Solid Edge part; units mm, degrees
sketch "Sketch1" plane through (0, 0, 0) normal (0, 0, 1) x (1, 0, 0)
  line L0 (-3, -3) -> (3, -3)
  line L1 (3, -3) -> (3, 3)
  line L2 (3, 3) -> (-3, 3)
  line L3 (-3, 3) -> (-3, -3)
extrude "Protrusion1" add sketch "Sketch1" along normal blind 2.5
sketch "Sketch2" plane through (0, 0, 2.5) normal (0, 0, 1) x (1, 0, 0)
  circle A0 centre (0, 0) radius 1
extrude "ExtrudedCutout_2" cut sketch "Sketch2" against normal blind 1
properties material "ABS Plastic, high impact"
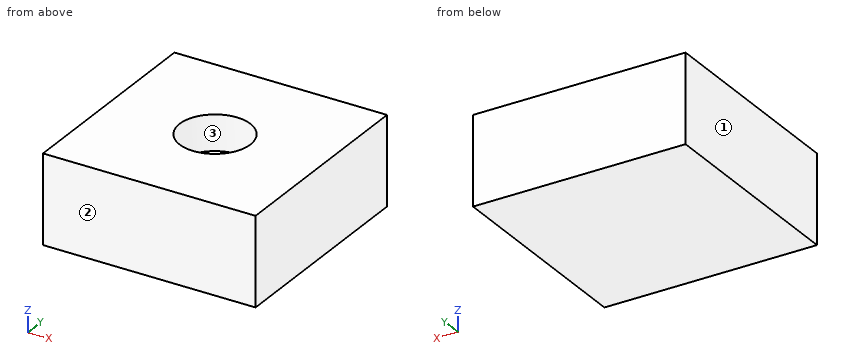
Work out the finished part from the listing and answer in its coordinate system (mm). Face numbers are marked on the shaded views. Give positions to 0.01 mm unless a question says otherwise; leave off trailing zeros. Order: outer loops, then holes, each group sorted by start corner. A loop starts at its lowest first (then second) coordinate and runs counter-clockwise, first axis right, second up. Notation, with made-up numbers: M -24.75,-7.75 L -1.75,-7.75 A21 cw -1.75,2.25 Z; hole C 83.25,52 d1. An arc over 180 degrees is marked long. Return JSON: item names as keys, results as strings.
1) Straight lines are drawn through the part: line 1 along Y through (x, z) = (0, 1.9); line 2 along X through (y, z) = (0.4, 1.75); line 3 along X through (y, z) = (0.7, 2.3). For each, find the intervals that lie inside material, in ascending order. Write a range as [from, to].
Resolved:
{"line 1": "[-3, -1], [1, 3]", "line 2": "[-3, -0.92], [0.92, 3]", "line 3": "[-3, -0.71], [0.71, 3]"}
2) For a pull along X with two mould halves and no side action, classify the marked faces 1, 2 and 3 as +X half, -X half, draft (parallel to the pull), parting line (faces both ways), or undercut.
Resolved:
{"face 1": "-X half", "face 2": "draft", "face 3": "undercut"}
3) Section A-A, the plane y = 0 is taken. Write down the section's boundary in (x, z), plus the area to 3 significant figures.
Resolved:
{"outline": "M -3,0 L 3,0 L 3,2.5 L 1,2.5 L 1,1.5 L -1,1.5 L -1,2.5 L -3,2.5 Z", "area": "13.0 mm^2"}
4) Each of these flat-tipped pins is pushed along its axis until it touches: pin 1 (1 mm diameter, centred on x = 0, y = 0, fed in from +Z); pin 2 (2.5 mm diameter, centred on x = 0, y = 0, fed in from +Z). Where does it stop, or does it pass through?
Resolved:
{"pin 1": "z = 1.5", "pin 2": "z = 2.5"}
5) Section B-B, the plane z = 2.35 is taken. Write down the section's boundary in (x, y), plus the area to 3 significant figures.
Resolved:
{"outline": "M -3,-3 L 3,-3 L 3,3 L -3,3 Z; hole C 0,0 d2", "area": "32.9 mm^2"}
